Can you work these out from the model? Positions are in its coordinate system, mm. A direction names the side the tool comes from. Coordinates: 2 decimals unless noted, no trailing zeros. Loops run counter-clockwise (first coordinate to the right, second up) from the corner with the lowest first, then second, coordinate; pieces in that order, holes last. Notation, with made-up numbers: M 75.5,75.5 L 106.5,75.5 A28 ccw 106.5,111.5 Z; hole C 59.5,-6.75 d1. An arc over 180 degrees is marked long. Answer as a JSON object with one key per item and string values. Group by question number.
Item 1: I'm going to push flat-ended pins straight in: pin 1 Ø0.5 at (x, z) = (-5.5, -0.5) entering from -Y; pin 2 Ø1.1 at (x, z) = (8, -0.5) entering from +Y; pin 3 Ø3 at (x, y) = (2.6, -50.2) entering from -Z; pin 4 Ø1.8 at (x, y) = (0.63, -55.44) entering from -Z. Where does each tip first touch, or does it pass through?
Item 2: Suppose I cut it at C-C (z = -1.25). Write out the boundary of the cut face in (x, y).
Item 3: If I drill on line 1 (Y direction, x = 1, z = -1.75); line 2 (Z direction, x = 3.5, y = -48.25); line 3 (X direction, y = -56.75, z = -0.65), over which ranges is the centre line in solid material (lowest first)?
Item 4: We'd pull the mould along X, two halves only. Please class faces 5 (the flat face through (9, -48.2, -0.5)), 6 (the flat face through (-9, -45.8, -0.5)), 7 (the cylindrical face through (1.92, -56.2, -0.49)), 8 (the flat face through (-6, -63.4, -0.9)): +X half, -X half, draft (parallel to the pull), parting line (faces both ways), or undercut.
Item 5: Suppose I cut it at D-D (x = 6.25). Write out the boundary of the cut face in (y, z), then the cut area to 3 significant figures.
Item 6: Suppose I cut it at B-B (y = -59.5). Write out the boundary of the cut face in (x, z).
Item 7: Which directions (+Z, -Z, +X, -X, +Y, -Y) give clear straight access to the entire face, cutting with the end or side of a thin tool? Please do faces 1 (the flat face through (-6.005, -61.853, -1.507)), 2 (the flat face through (-6.4, -50.2, -0.5)), 3 (the cylindrical face through (-3.669, -58.844, -0.493)), 4 (the flat face through (-4.526, -62, -1)).
Item 8: Suppose I cut it at A-A (x = -2.6). Write out the boundary of the cut face in (y, z).
```python
from build123d import *

# Parameters (mm, degrees)
SKETCH_W             = 56
SKETCH_H             = 12
PAD_DEPTH            = 64
POCKET_DEPTH         = 8
PAD001_DEPTH         = 4.5
SKETCH005_R          = 2
SKETCH005_W          = 30
SKETCH005_H          = 5
POCKET001_DEPTH      = 10.5
SKETCH007_R          = 4
SKETCH007_W          = 3
SKETCH007_H          = 7
POCKET002_DEPTH      = 3
CHAMFER_SIZE         = 1.5
PAD002_DEPTH         = 2
CHAMFER001_SIZE      = 1.5
POCKET003_DEPTH      = 9.02746
POCKET003_DEPTH_BACK = 9.001


with BuildPart() as body003:
    # Sketch → Pad (new body)
    with BuildSketch(Plane.XZ):
        with Locations((0, -6)):
            Rectangle(SKETCH_W, SKETCH_H)
    extrude(amount=PAD_DEPTH)

    # Sketch002 → Pocket (cut)
    with BuildSketch(Plane.XY):
        Polygon((-24.2, 0), (-24.2, -57.2), (-17.9, -57.2), (-17.9, -39.2), (17.9, -39.2), (17.9, -57.2), (24.2, -57.2), (24.2, 0), align=None)
        with BuildLine():
            Line((-9, -41.2), (-9, -50.2))
            Line((-9, -50.2), (-3.7, -50.2))
            ThreePointArc((-1.5, -50.2), (-2.6, -49.1), (-3.7, -50.2))
            ThreePointArc((-1.5, -50.2), (-0.771185, -52.533477), (1.156153, -54.037357))
            ThreePointArc((-0.285678, -56.630951), (1.938949, -56.170097), (1.156153, -54.037357))
            ThreePointArc((-0.285678, -56.630951), (-5.015993, -56.163695), (-7.52646, -60.2))
            Line((-7.52646, -60.2), (-7.52646, -67.774911))
            Line((-7.52646, -67.774911), (-4.52646, -67.774911))
            Line((-4.52646, -67.774911), (-4.52646, -60.2))
            ThreePointArc((-2.112866, -59.010317), (-3.689638, -58.854565), (-4.52646, -60.2))
            ThreePointArc((-2.112866, -59.010317), (4.561015, -57.627756), (2.212626, -51.229535))
            ThreePointArc((3.7, -50.2), (1.973945, -49.295536), (2.212626, -51.229535))
            Line((9, -50.2), (3.7, -50.2))
            Line((9, -46.2), (9, -50.2))
            Line((6, -46.2), (9, -46.2))
            Line((6, -41.2), (6, -46.2))
            Line((-9, -41.2), (6, -41.2))
        make_face()
    extrude(amount=-POCKET_DEPTH, mode=Mode.SUBTRACT)

    # Sketch006 → Pad001 (join)
    with BuildSketch(Plane.XY):
        Polygon((-25.2, -12), (-22.614214, -12), (-21.2, -13.414214), (-21.2, -58), (-25.2, -58), align=None)
        Polygon((25.2, -12), (22.614214, -12), (21.2, -13.414214), (21.2, -58), (25.2, -58), align=None)
    extrude(amount=-PAD001_DEPTH)

    # Sketch005 → Pocket001 (cut)
    with BuildSketch(Plane.XY):
        with Locations((-12.5, -56)):
            Circle(SKETCH005_R)
        with Locations((12.5, -56)):
            Circle(SKETCH005_R)
        with BuildLine():
            Line((-12.25, -29), (-12.25, -49.5))
            Line((-12.25, -49.5), (-3.75, -49.5))
            Line((-3.75, -49.5), (-3.75, -49))
            Line((-3.75, -49), (-11.25, -49))
            ThreePointArc((-11.75, -48.5), (-11.603553, -48.853553), (-11.25, -49))
            Line((-11.75, -48.5), (-11.75, -29))
            Line((-11.75, -29), (-12.25, -29))
        make_face()
        with BuildLine():
            Line((12.25, -29), (12.25, -49.5))
            Line((12.25, -49.5), (3.75, -49.5))
            Line((3.75, -49.5), (3.75, -49))
            Line((3.75, -49), (11.25, -49))
            ThreePointArc((11.25, -49), (11.603553, -48.853553), (11.75, -48.5))
            Line((11.75, -48.5), (11.75, -29))
            Line((11.75, -29), (12.25, -29))
        make_face()
        with Locations((0, -6.3)):
            Rectangle(SKETCH005_W, SKETCH005_H)
    extrude(amount=-POCKET001_DEPTH, mode=Mode.SUBTRACT)

    # Sketch007 → Pocket002 (cut)
    with BuildSketch(Plane.XY):
        with Locations((-12.5, -56)):
            Circle(SKETCH007_R)
        with Locations((12.5, -56)):
            Circle(SKETCH007_R)
        with Locations((8.5, -41.5)):
            Rectangle(SKETCH007_W, SKETCH007_H)
    extrude(amount=-POCKET002_DEPTH, mode=Mode.SUBTRACT)

    # Chamfer
    chamfer_edges = [body003.edges().sort_by_distance(p)[0] for p in [
        (28, -32, -12),
        (-28, -32, -12),
        (0, 0, -12),
        (0, -64, -12),
        (28, -32, 0),
        (28, 0, -6),
        (28, -64, -6),
        (-28, -32, 0),
        (-28, 0, -6),
        (-28, -64, -6),
        (11.73677, -64, 0),
        (-4.52646, -64, -4),
        (-6.02646, -64, -8),
        (-7.52646, -64, -4),
        (-17.76323, -64, 0),
        (-26.1, 0, 0),
        (26.1, 0, 0),
    ]]
    chamfer(chamfer_edges, length=CHAMFER_SIZE)


with BuildPart() as cablecover:
    # Sketch008 → Pad002 (new body)
    with BuildSketch(Plane.XY):
        Polygon((5.266473, -64), (-9.544278, -64), (-7.665841, -56.897079), (-9, -50.2), (-9, -41.2), (6.447607, -41.2), (6.447607, -45.58699), (9, -45.58699), (9, -50.2), align=None)
    extrude(amount=-PAD002_DEPTH)

    # Chamfer001
    chamfer001_edges = [cablecover.edges().sort_by_distance(p)[0] for p in [
        (-2.138902, -64, 0),
    ]]
    chamfer(chamfer001_edges, length=CHAMFER001_SIZE)

    # Cut: cut Body003
    add(body003.part, mode=Mode.SUBTRACT)

    # Sketch009 → Pocket003 (cut, two sides)
    with BuildSketch(Plane.YZ) as pocket003_sk:
        Polygon((-42.730701, -2), (-62.409084, -2), (-61.282127, -1), (-42.730701, -1), align=None)
    extrude(amount=-POCKET003_DEPTH, mode=Mode.SUBTRACT)
    extrude(pocket003_sk.sketch, amount=POCKET003_DEPTH_BACK, mode=Mode.SUBTRACT)


solid = cablecover.part
```
From the geometry:
{
 "1": {"pin 1": "y = -63.25", "pin 2": "y = -46.2", "pin 3": "z = -1", "pin 4": "through"},
 "2": {"outline": "M -9,-42.73 L 6,-42.73 L 6,-41.2 L -9,-41.2 Z; M -8.78,-63.75 L -3.28,-63.75 L -4.53,-62.5 L -4.53,-61.56 L -7.53,-61.56 L -7.53,-62.5 Z"},
 "3": {"line 1": "-42.73 to -41.2", "line 2": "-1 to 0", "line 3": "-5.92 to -0.11, 1.36 to 4.93"},
 "4": {"face 5": "+X half", "face 6": "-X half", "face 7": "undercut", "face 8": "draft"},
 "5": {"outline": "M -50.2,-1 L -46.2,-1 L -46.2,0 L -50.2,0 Z", "area": "4.00 mm2"},
 "6": {"outline": "M -7.47,-1 L -4.35,-1 L -4.35,0 L -7.47,0 Z; M -1.32,-1 L 2.57,-1 L 2.57,0 L -1.32,0 Z"},
 "7": {"face 1": "-Z, +X, -X", "face 2": "+Z, -Z, -X", "face 3": "+Z, -Z", "face 4": "+Z, -Z, +X"},
 "8": {"outline": "M -58.76,-1 L -55.72,-1 L -55.72,0 L -58.76,0 Z; M -49.1,-1 L -42.73,-1 L -42.73,-2 L -41.2,-2 L -41.2,0 L -49.1,0 Z"}
}
